Design review of the part built by this model. Coordinates are the model's own, in mm. Give positions to 0.01 mm unless a question says otherwise; leave off trailing zeros. Order: outer loops, then holes, each group sorted by start corner. A loop starts at its lowest first (then second) coordinate and runs counter-clockwise, first axis right, second up. Notation, with made-up numbers: (37.25, 57.5) -> (85.25, 57.5) arc R32 ccw to (85.25, 96.5) -> close; hole circle Ø4 at (28.5, -34.5). An arc over 180 degrees is marked (long way). One line per item, written item: value.
from build123d import *

# Parameters (mm, degrees)
F0_R     = 2.5
F0_R_2   = 1.15
F1_DEPTH = 1
F2_W     = 15
F2_H     = 15
F2_R     = 5
F2_R_2   = 2.5
F2_R_3   = 1.15
F3_DEPTH = 1
F4_R     = 3
F6_W     = 15
F6_H     = 35
F6_R     = 1.5
F6_R_2   = 1.15
F7_DEPTH = 1
F8_R     = 7


# Not quite as in the source:
# - a feature of the source that left no trace in its solid (it failed there, or was rolled back) is left out


with BuildPart() as f1:
    # F0 (on Top) → F1 (new body)
    with BuildSketch(Plane.XY):
        Circle(F0_R)
        Circle(F0_R_2, mode=Mode.SUBTRACT)
    extrude(amount=F1_DEPTH)

    # F2 (on face) → F3 (join)
    with BuildSketch(Plane(origin=(0, 0, 0), x_dir=(1, 0, 0), z_dir=(0, 0, -1))):
        Rectangle(F2_W, F2_H)
        Circle(F2_R, mode=Mode.SUBTRACT)
        Circle(F2_R)
        Circle(F2_R_2, mode=Mode.SUBTRACT)
        Circle(F2_R_2)
        Circle(F2_R_3, mode=Mode.SUBTRACT)
    extrude(amount=F3_DEPTH)

    # F4
    f4_edges = [f1.edges().sort_by_distance(p)[0] for p in [
        (-7.5, 7.5, -0.5),
        (7.5, 7.5, -0.5),
        (-7.5, -7.5, -0.5),
        (7.5, -7.5, -0.5),
    ]]
    fillet(f4_edges, radius=F4_R)

    # F6 (on face) → F7 (join)
    with BuildSketch(Plane.XY):
        Rectangle(F6_W, F6_H)
        with Locations((0, -14)):
            Circle(F6_R, mode=Mode.SUBTRACT)
        Circle(F6_R_2, mode=Mode.SUBTRACT)
        with Locations((0, 14)):
            Circle(F6_R, mode=Mode.SUBTRACT)
    extrude(amount=F7_DEPTH)

    # F8
    f8_edges = [f1.edges().sort_by_distance(p)[0] for p in [
        (-7.5, 17.5, 0.5),
        (7.5, 17.5, 0.5),
        (7.5, -17.5, 0.5),
        (-7.5, -17.5, 0.5),
    ]]
    fillet(f8_edges, radius=F8_R)


solid = f1.part
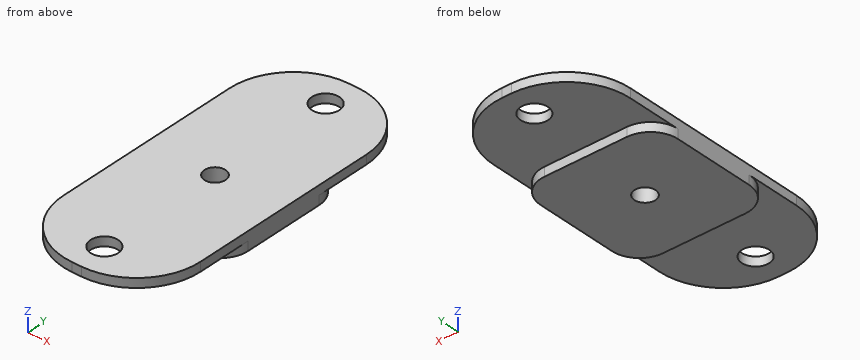
Item 1: To check wall thickness, follow line 1 along Y through (x, z) = (0, 0.35); line 2 along X through (y, z) = (0, -0.1); line 3 along Y through (x, z) = (-4, -0.7). State the ranges of each line that lie inside material, in increasing order. Write a range as from..to.
Returned:
line 1: -17.5..-15.5, -12.5..-1.15, 1.15..12.5, 15.5..17.5
line 2: -7.5..-1.15, 1.15..7.5
line 3: -7.5..7.5
Item 2: Add section C-C on x = 0. Give the boundary of the cut face in (y, z).
Returned:
outline: (-17.5, 0) -> (-15.5, 0) -> (-15.5, 1) -> (-17.5, 1) -> close; (-12.5, 0) -> (-7.5, 0) -> (-7.5, -1) -> (-1.15, -1) -> (-1.15, 1) -> (-12.5, 1) -> close; (1.15, -1) -> (7.5, -1) -> (7.5, 0) -> (12.5, 0) -> (12.5, 1) -> (1.15, 1) -> close; (15.5, 0) -> (17.5, 0) -> (17.5, 1) -> (15.5, 1) -> close
Item 3: Add section B-B on z = -0.35. Give the boundary of the cut face in (x, y).
Returned:
outline: (-7.5, -4.5) arc R3 ccw to (-4.5, -7.5) -> (4.5, -7.5) arc R3 ccw to (7.5, -4.5) -> (7.5, 4.5) arc R3 ccw to (4.5, 7.5) -> (-4.5, 7.5) arc R3 ccw to (-7.5, 4.5) -> close; hole circle Ø2.3 at (0, 0)
Item 4: Add section D-D on y = -14. Give the boundary of the cut face in (x, z).
Returned:
outline: (-6.56, 0) -> (-1.5, 0) -> (-1.5, 1) -> (-6.56, 1) -> close; (1.5, 0) -> (6.56, 0) -> (6.56, 1) -> (1.5, 1) -> close
Item 5: Clearance check with flat-ended pins moving along their axes: P1, Ø0.8, axis at x = 0, z = -0.5, coming from the +Y side; P2, Ø6.5, axis at x = -3, y = 12, coming from the -Z side; P3, Ø0.8, axis at x = -2, z = -0.5, coming from the -Y side. State where each tip first meets the part, or that it passes through.
Returned:
P1: y = 7.5
P2: z = 0
P3: y = -7.5
Item 6: Add section A-A on y = 0. Give the boundary of the cut face in (x, z).
Returned:
outline: (-7.5, -1) -> (-1.15, -1) -> (-1.15, 1) -> (-7.5, 1) -> close; (1.15, -1) -> (7.5, -1) -> (7.5, 1) -> (1.15, 1) -> close
